Geometry: final body of the model. Coordinates: model frame, mm. Give positions to 0.01 mm unless a question says otherwise; leave off trailing zeros. Write each loop counter-clockwise with the first axis right and the second up, starting at its lowest first coordinate (ties: lowest second). Pieces come first, ordered by that corner, then holes.
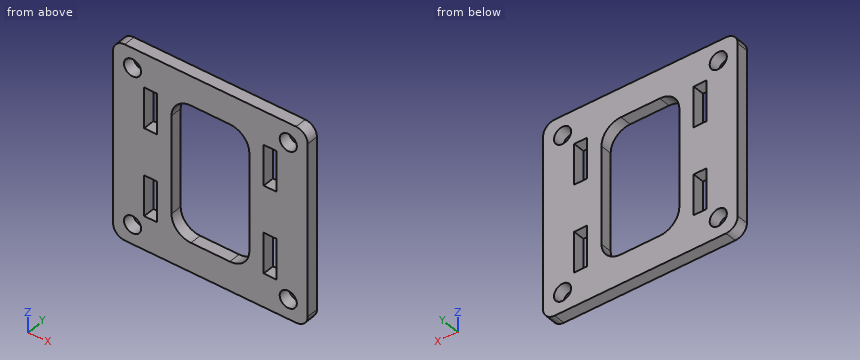
from build123d import *

# Parameters (mm, degrees)
SKETCH_1_W          = 50
SKETCH_1_H          = 50
SKETCH_1_W_2        = 3.3
SKETCH_1_H_2        = 10.4
EXTRUDE_1_DEPTH     = 3
SKETCH_2_W          = 20
SKETCH_2_H          = 35
CUT_EXTRUDE_1_DEPTH = 3
FILLET_1_R          = 5
SKETCH_3_R          = 2.2
CUT_EXTRUDE_2_DEPTH = 3
FILLET_2_R          = 3


with BuildPart() as part:
    # 草图1 → 凸台-拉伸1 (new body)
    with BuildSketch(Plane(origin=(0, 0, 0), x_dir=(1, 0, 0), z_dir=(0, 1, 0))):
        Rectangle(SKETCH_1_W, SKETCH_1_H)
        with Locations((15.35, 11.2)):
            Rectangle(SKETCH_1_W_2, SKETCH_1_H_2, mode=Mode.SUBTRACT)
        with Locations((15.35, -11.2)):
            Rectangle(SKETCH_1_W_2, SKETCH_1_H_2, mode=Mode.SUBTRACT)
        with Locations((-15.35, -11.2)):
            Rectangle(SKETCH_1_W_2, SKETCH_1_H_2, mode=Mode.SUBTRACT)
        with Locations((-15.35, 11.2)):
            Rectangle(SKETCH_1_W_2, SKETCH_1_H_2, mode=Mode.SUBTRACT)
    extrude(amount=EXTRUDE_1_DEPTH)

    # 草图2 → 切除-拉伸1 (cut)
    with BuildSketch(Plane(origin=(0, 3, 0), x_dir=(1, 0, 0), z_dir=(0, 1, 0))):
        Rectangle(SKETCH_2_W, SKETCH_2_H)
    extrude(amount=-CUT_EXTRUDE_1_DEPTH, mode=Mode.SUBTRACT)

    # 圆角1
    fillet_1_edges = [part.edges().sort_by_distance(p)[0] for p in [
        (10, 1.5, -17.5),
        (10, 1.5, 17.5),
        (-10, 1.5, 17.5),
        (-10, 1.5, -17.5),
    ]]
    fillet(fillet_1_edges, radius=FILLET_1_R)

    # 草图3 → 切除-拉伸2 (cut)
    with BuildSketch(Plane(origin=(0, 3, 0), x_dir=(1, 0, 0), z_dir=(0, 1, 0))):
        with Locations(Location((-20, 20, 0), (0, 0, 270))):
            Circle(SKETCH_3_R)
        with Locations(Location((20, 20, 0), (0, 0, 270))):
            Circle(SKETCH_3_R)
        with Locations(Location((20, -20, 0), (0, 0, 270))):
            Circle(SKETCH_3_R)
        with Locations(Location((-20, -20, 0), (0, 0, 270))):
            Circle(SKETCH_3_R)
    extrude(amount=-CUT_EXTRUDE_2_DEPTH, mode=Mode.SUBTRACT)

    # 圆角2
    fillet_2_edges = [part.edges().sort_by_distance(p)[0] for p in [
        (25, 1.5, 25),
        (-25, 1.5, 25),
        (-25, 1.5, -25),
        (25, 1.5, -25),
    ]]
    fillet(fillet_2_edges, radius=FILLET_2_R)


solid = part.part
Q1. Pin query (flat end, axial travel): P1, Ø12, axis at x = 10.5, z = -14.5, coming from the -Y side. Return the tip coordinate at first contact, or that it passes through.
Filled sheet:
P1: stops at y = 0
Q2. Ray query, line 1 along Z through (x, y) = (-14, 1); line 2 along X through (y, z) = (1.7, 20); line 3 along X through (y, z) = (1.75, 4). Return the intervals inside material, ascending.
Filled sheet:
line 1: z = -25 to -16.4, -6 to 6, 16.4 to 25
line 2: x = -25 to -22.2, -17.8 to 17.8, 22.2 to 25
line 3: x = -25 to -10, 10 to 25
Q3. Section D-D on z = 9.5. Output: boundary loops of the cut face in (x, y).
Filled sheet:
outline: (-25, 0) - (-17, 0) - (-17, 3) - (-25, 3) - close; (-13.7, 0) - (-10, 0) - (-10, 3) - (-13.7, 3) - close; (10, 0) - (13.7, 0) - (13.7, 3) - (10, 3) - close; (17, 0) - (25, 0) - (25, 3) - (17, 3) - close
Q4. Section A-A on x = -14.5. Output: boundary loops of the cut face in (y, z).
Filled sheet:
outline: (0, -25) - (3, -25) - (3, -16.4) - (0, -16.4) - close; (0, -6) - (3, -6) - (3, 6) - (0, 6) - close; (0, 16.4) - (3, 16.4) - (3, 25) - (0, 25) - close
Q5. Section C-C on x = 2. Output: boundary loops of the cut face in (y, z), plus the area to 3 significant figures.
Filled sheet:
outline: (0, -25) - (3, -25) - (3, -17.5) - (0, -17.5) - close; (0, 17.5) - (3, 17.5) - (3, 25) - (0, 25) - close
area: 45.0 mm2
Q6. Section B-B on z = -20. Output: boundary loops of the cut face in (x, y), plus the area to 3 significant figures.
Filled sheet:
outline: (-25, 0) - (-22.2, 0) - (-22.2, 3) - (-25, 3) - close; (-17.8, 0) - (17.8, 0) - (17.8, 3) - (-17.8, 3) - close; (22.2, 0) - (25, 0) - (25, 3) - (22.2, 3) - close
area: 124 mm2
